Geometry check sheet. Reference: the model listing, model coordinates, mm. Face numbers are marked on the shaded views. A direction names the side the tool comes from. Give positions to 0.01 mm unless a question says otherwise; leave off trailing zeros. Write each loop counter-clockwise with the first axis right and the second up, starting at its lowest first coordinate (ties: lowest second). Pieces come first, ordered by that corner, then holes. Notation, with made-up numbers: (59.5, 87.25) - (88.5, 87.25) arc R32 cw to (88.5, 121.25) - close; hole circle Ø9 at (-39, -26.5). An arc over 180 degrees is marked (long way). One line per question, with ' | ' between items. Start each with the question number.
Q1. Section check C-C on z = 6. Record the boundary of the cut face in (x, y).
Q2. Section check B-B on x = 22. Record the boundary of the cut face in (y, z), and give its area (4 significant figures).
Q3. Gauge pin test, flat ends, axial feed: P1, Ø1.8, axis at x = 28, y = 0.5, coming from the +Z side; P2, Ø3.5, axis at y = 3.5, z = 6.5, coming from the -X side; P3, Ø2.5, axis at y = 6, z = 4, coming from the -X side; P4, Ø2.5, axis at x = -28.5, y = 0, coming from the +Z side. Record the tip position at first contact, or that the pin passes through.
Q4. Section check A-A on y = 0. Record the boundary of the cut face in (x, z), and give its area (3 significant figures).
Q5. Release check for a two-part mould opening along Z. For the marked faces 1, 2 and 3 record: +Z half, -Z half, draft (parallel to the pull), parting line (faces both ways), or undercut.
Q6. Thickness scan on L1, parallel to X at y = 0, z = 1.4; L2, parallel to Z at x = 3.5, y = 0.5; L3, parallel to X at y = -4.75, z = 3.75. Record the ranges inside material, lowest first. Write a range as [from, to].
Q7. Set-up check for the marked faces 4, 5 and 6: record each of +Z, -Z, +X, -X, +Y, -Y from which the full face is reachable in a straight line by a thin tool's end or side.
```python
from build123d import *

# Parameters (mm, degrees)
SKETCH1_W               = 55
SKETCH1_H               = 21
BOSS_EXTRUDE1_DEPTH     = 12
SHELL1_T                = -2.5
SKETCH2_R               = 3
BOSS_EXTRUDE2_DEPTH     = 3
CUT_EXTRUDE1_DEPTH      = 30
CUT_EXTRUDE1_DEPTH_BACK = 5
SKETCH3_R               = 1.5
CUT_EXTRUDE5_START      = -9
SKETCH4_R               = 3
CUT_EXTRUDE5_DEPTH      = 9
FILLET1_DEPTH           = 3


with BuildPart() as part:
    # Sketch1 → Boss-Extrude1 (new body)
    with BuildSketch(Plane.XY):
        Rectangle(SKETCH1_W, SKETCH1_H)
    extrude(amount=BOSS_EXTRUDE1_DEPTH)

    # Shell1
    shell1_openings = [part.faces().sort_by_distance(p)[0] for p in [
        (0, 10.5, 6),
    ]]
    offset(amount=SHELL1_T, openings=shell1_openings, kind=Kind.INTERSECTION)

    # Sketch2 → Boss-Extrude2 (add)
    with BuildSketch(Plane(origin=(0, 0, 0), x_dir=(-1, 0, 0), z_dir=(0, 0, -1))):
        with Locations((28.5, 0)):
            Circle(SKETCH2_R)
        with Locations((-28.5, 0)):
            Circle(SKETCH2_R)
    extrude(amount=-BOSS_EXTRUDE2_DEPTH)

    # Sketch3 → Cut-Extrude1 (cut, two sides: drawn at the far end of the back side and taken through both)
    with BuildSketch(Plane.XY.offset(3).offset(-CUT_EXTRUDE1_DEPTH_BACK)):
        with Locations(Location((-28.5, 0, 0), (0, 0, 48.189685104))):
            Circle(SKETCH3_R)
        with Locations(Location((28.5, 0, 0), (0, 0, 131.810314896))):
            Circle(SKETCH3_R)
    extrude(amount=CUT_EXTRUDE1_DEPTH + CUT_EXTRUDE1_DEPTH_BACK, mode=Mode.SUBTRACT)

    # Sketch4 → Cut-Extrude5 (cut)
    with BuildSketch(Plane.XY.offset(12).offset(CUT_EXTRUDE5_START)):
        with Locations((-28.5, 0)):
            Circle(SKETCH4_R)
        with Locations((28.5, 0)):
            Circle(SKETCH4_R)
    extrude(amount=CUT_EXTRUDE5_DEPTH, mode=Mode.SUBTRACT)

    # Fillet1: read off the stored shape, not the designer's step
    # Fillet1 outline → Fillet1 (add)
    with BuildSketch(Plane.XY):
        with BuildLine():
            add(Edge.make_bspline(
                [(30, -2.598076211), (29.735280722, -2.750911958), (29.325654839, -2.942455607), (28.108593688, -3.775872627), (27.622600662, -4.829914939), (27.5, -5.892304845), (27.5, -6.410254038), (27.5, -6.92820323)],
                knots=[0, 0, 0, 0, 0, 0, 0.5, 0.5, 1, 1, 1, 1, 1, 1], degree=5))
            ThreePointArc((30, -2.598076211), (28.775255129, -2.987345748), (27.5, -2.828427125))
            Line((27.5, -2.828427125), (27.5, -6.92820323))
        make_face()
        with BuildLine():
            add(Edge.make_bspline(
                [(27.5, 6.92820323), (27.5, 6.410254038), (27.5, 5.892304845), (27.622600662, 4.829914939), (28.108593688, 3.775872627), (29.325654839, 2.942455607), (29.735280722, 2.750911958), (30, 2.598076211)],
                knots=[0, 0, 0, 0, 0, 0, 0.5, 0.5, 1, 1, 1, 1, 1, 1], degree=5))
            Line((27.5, 6.92820323), (27.5, 2.828427125))
            ThreePointArc((27.5, 2.828427125), (28.775255129, 2.987345748), (30, 2.598076211))
        make_face()
        with BuildLine():
            add(Edge.make_bspline(
                [(-30, 2.598076211), (-29.735280722, 2.750911958), (-29.325654839, 2.942455607), (-28.108593688, 3.775872627), (-27.622600662, 4.829914939), (-27.5, 5.892304845), (-27.5, 6.410254038), (-27.5, 6.92820323)],
                knots=[0, 0, 0, 0, 0, 0, 0.5, 0.5, 1, 1, 1, 1, 1, 1], degree=5))
            ThreePointArc((-30, 2.598076211), (-28.775255129, 2.987345748), (-27.5, 2.828427125))
            Line((-27.5, 2.828427125), (-27.5, 6.92820323))
        make_face()
        with BuildLine():
            add(Edge.make_bspline(
                [(-27.5, -6.92820323), (-27.5, -6.410254038), (-27.5, -5.892304845), (-27.622600662, -4.829914939), (-28.108593688, -3.775872627), (-29.325654839, -2.942455607), (-29.735280722, -2.750911958), (-30, -2.598076211)],
                knots=[0, 0, 0, 0, 0, 0, 0.5, 0.5, 1, 1, 1, 1, 1, 1], degree=5))
            Line((-27.5, -6.92820323), (-27.5, -2.828427125))
            ThreePointArc((-27.5, -2.828427125), (-28.775255129, -2.987345748), (-30, -2.598076211))
        make_face()
    extrude(amount=FILLET1_DEPTH)


solid = part.part
```
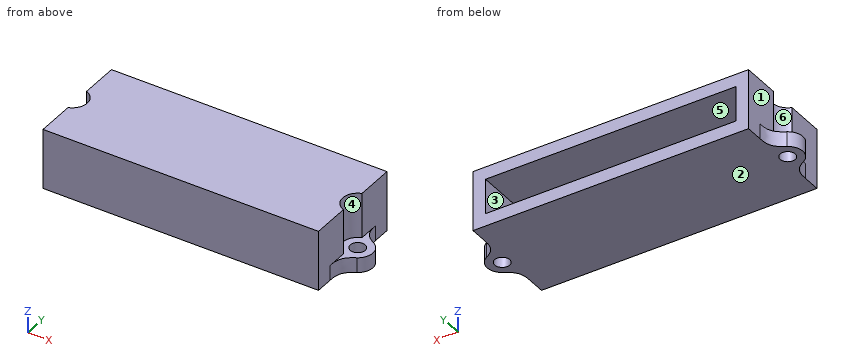
Working result:
1) outline: (-27.5, -10.5) - (27.5, -10.5) - (27.5, -2.83) arc R3 cw to (27.5, 2.83) - (27.5, 10.5) - (25, 10.5) - (25, -8) - (-25, -8) - (-25, 10.5) - (-27.5, 10.5) - (-27.5, 2.83) arc R3 cw to (-27.5, -2.83) - close
2) outline: (-10.5, 0) - (10.5, 0) - (10.5, 2.5) - (-8, 2.5) - (-8, 9.5) - (10.5, 9.5) - (10.5, 12) - (-10.5, 12) - close | area: 122.5 mm2
3) P1: stops at z = 3 | P2: stops at x = -27.5 | P3: stops at x = -27.64 | P4: passes through
4) outline: (-31.5, 0) - (-30, 0) - (-30, 3) - (-31.5, 3) - close; (-27, 0) - (27, 0) - (27, 3) - (25.5, 3) - (25.5, 12) - (-25.5, 12) - (-25.5, 3) - (-27, 3) - close; (30, 0) - (31.5, 0) - (31.5, 3) - (30, 3) - close; hole (-25, 2.5) - (25, 2.5) - (25, 9.5) - (-25, 9.5) - close | area: 280 mm2
5) face 1: draft | face 2: -Z half | face 3: undercut
6) L1: x = [-31.5, -30], [-27, 27], [30, 31.5] | L2: z = [0, 2.5], [9.5, 12] | L3: x = [-27.5, -25], [25, 27.5]
7) face 4: +Z, +X | face 5: +Y | face 6: +Z, -X
